Can you work these out from the drawing? Everything is in mm from the part's minimum corner. A direction names the side the tool comes from. Coordinates: 2 decimals unless noted, no trailing zeros. Loops run counter-clockwise (first coordinate to the right, second up) from the corner with the lowest first, then second, coordinate; pieces in that order, holes last.
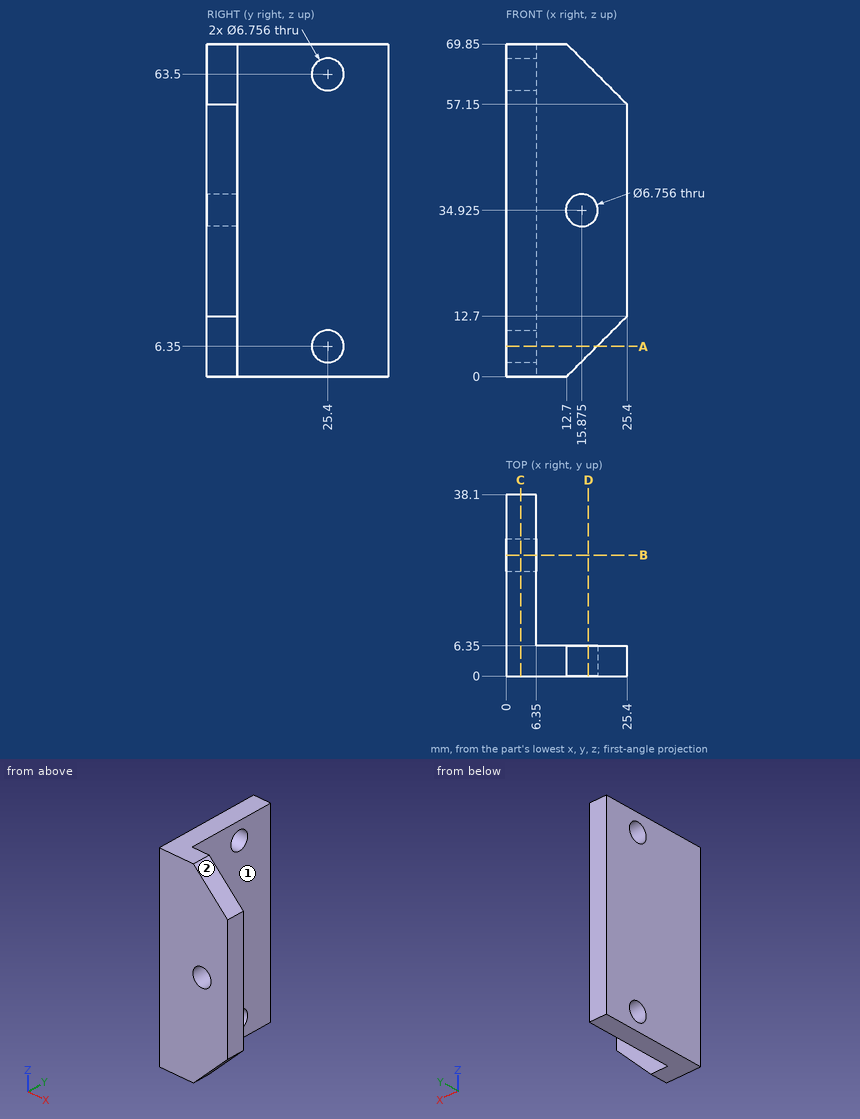
(1) Imagine slicing it at D-D, the plane x = 17.25. Write out the boundary of the cut face in (y, z).
Answers:
outline: (0, 4.55) - (6.35, 4.55) - (6.35, 31.84) - (0, 31.84) - close; (0, 38.01) - (6.35, 38.01) - (6.35, 65.3) - (0, 65.3) - close
(2) I need wall thicknesses on probe 1 along Y at (x, z) = (3.25, 6.35); probe 2 along Y at (x, z) = (9.5, 15.5); probe 3 along Z at (x, y) = (18.25, 4). Which ranges of each line are inside material? Lowest first, please.
Answers:
probe 1: y = 0 to 22.02, 28.78 to 38.1
probe 2: y = 0 to 6.35
probe 3: z = 5.55 to 32.52, 37.33 to 64.3
(3) Which directions (+Z, -Z, +X, -X, +Y, -Y) give clear straight access to the entire face, cutting with the end or side of a thin tool? Please do the marked faces 1 and 2.
Answers:
face 1: +Z, -Z, +X, +Y
face 2: +Z, +X, +Y, -Y
(4) For pin 1 (1 mm diameter, centred on y = 25, z = 62.5, fed in from +X); pin 2 (2 mm diameter, centred on x = 20, z = 48, fed in from +Y); pin 3 (16 mm diameter, centred on y = 18, z = 31.5, fed in from +X); pin 4 (8 mm diameter, centred on y = 25.4, z = 63.5, fed in from -X), each with a flat end and sliding along its axis, tell me the tip position at first contact or that it passes through.
Answers:
pin 1: passes through
pin 2: stops at y = 6.35
pin 3: stops at x = 6.35
pin 4: stops at x = 0
(5) Imagine slicing it at A-A, the plane z = 6.35. Write out the boundary of the cut face in (x, y), and give its area (3 significant figures).
Answers:
outline: (0, 0) - (19.05, 0) - (19.05, 6.35) - (6.35, 6.35) - (6.35, 22.02) - (0, 22.02) - close; (0, 28.78) - (6.35, 28.78) - (6.35, 38.1) - (0, 38.1) - close
area: 280 mm2
(6) Imagine slicing it at B-B, the plane y = 25.4. Write out the boundary of the cut face in (x, z).
Answers:
outline: (0, 0) - (6.35, 0) - (6.35, 2.97) - (0, 2.97) - close; (0, 9.73) - (6.35, 9.73) - (6.35, 60.12) - (0, 60.12) - close; (0, 66.88) - (6.35, 66.88) - (6.35, 69.85) - (0, 69.85) - close
(7) Imagine slicing it at C-C, the plane x = 3. Write out the boundary of the cut face in (y, z).
Answers:
outline: (0, 0) - (38.1, 0) - (38.1, 69.85) - (0, 69.85) - close; hole circle Ø6.76 at (25.4, 6.35); hole circle Ø6.76 at (25.4, 63.5)
